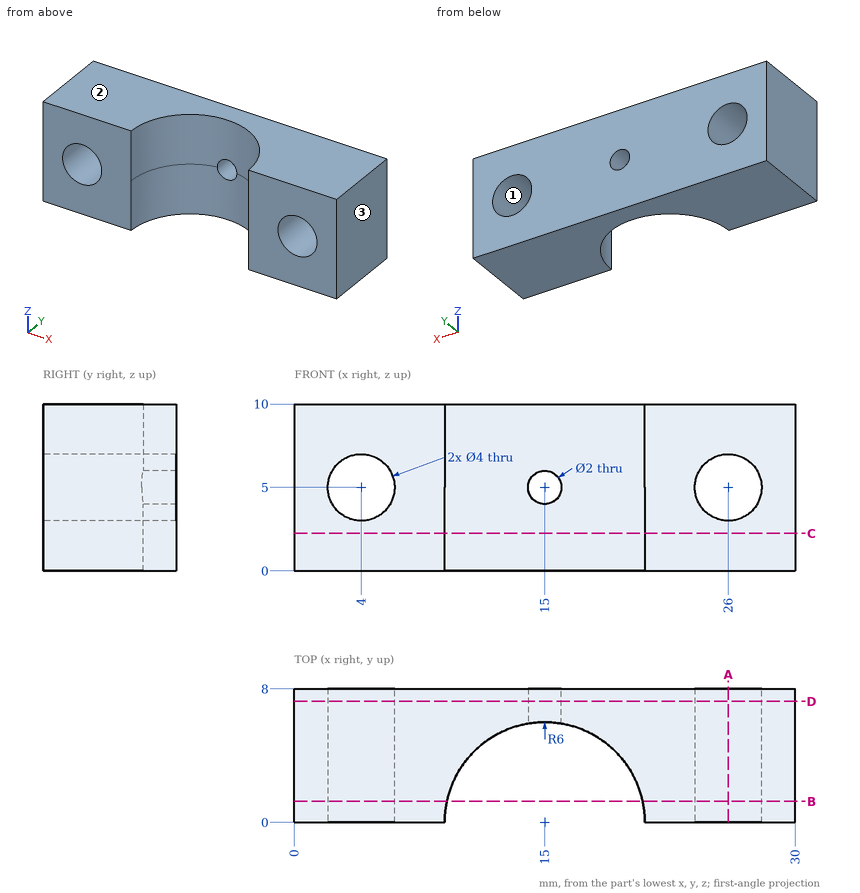
Part print with two shaded views. Sizes in mm from the minimum x, y, z corner. Round coordinates to 2 decimals unless told otherwise and drop trailing zeros. Write each loop counter-clockwise with the first axis right and the second up, starting at its lowest first coordinate (ties: lowest second). Pieces come first, ordered by that corner, then holes. Notation, with made-up numbers: (79, 64) -> (86, 64) arc R7 ccw to (86, 68) -> close; hole circle Ø1 at (84, -22). An arc over 180 degrees is marked (long way). Put each result on its own line as item: value.
Item 1: Wall check: probe 1 along Z at (x, y) = (26, 4.5); probe 2 along X at (y, z) = (6.5, 5.75); probe 3 along X at (y, z) = (7.25, 3.5). Give the ranges that are in metal, low to high. Write a range as from..to.
Here are the results:
probe 1: z = 0..3, 7..10
probe 2: x = 0..2.15, 5.85..14.34, 15.66..24.15, 27.85..30
probe 3: x = 0..2.68, 5.32..24.68, 27.32..30
Item 2: Slice it at B-B, the plane y = 1.25. Give the cut face in (x, z).
Here are the results:
outline: (0, 0) -> (9.13, 0) -> (9.13, 10) -> (0, 10) -> close; (20.87, 0) -> (30, 0) -> (30, 10) -> (20.87, 10) -> close; hole circle Ø4 at (4, 5); hole circle Ø4 at (26, 5)
Item 3: Slice it at C-C, the plane z = 2.25. Give the cut face in (x, y), plus the area to 3 significant figures.
Here are the results:
outline: (0, 0) -> (9, 0) arc R6 cw to (21, 0) -> (30, 0) -> (30, 8) -> (0, 8) -> close
area: 183 mm^2
Item 4: Flat gauge pin, fed straight in: P1, Ø2.5, axis at x = 15, z = 5, coming from the -Y side. Where does the tip first touch, or does it go through?
Here are the results:
P1: stops at y = 5.87
Item 5: Two-plate mould, pull along Z, no slides. Class the marked faces 1, 2 and 3: pulls with the +Z half, pulls with the -Z half, needs draft (parallel to the pull), parting line crosses it, or undercut.
Here are the results:
face 1: undercut
face 2: pulls with the +Z half
face 3: needs draft
Item 6: Slice it at D-D, the plane y = 7.25. Give the cut face in (x, z), plus the area to 3 significant figures.
Here are the results:
outline: (0, 0) -> (30, 0) -> (30, 10) -> (0, 10) -> close; hole circle Ø4 at (4, 5); hole circle Ø2 at (15, 5); hole circle Ø4 at (26, 5)
area: 272 mm^2
Item 7: Slice it at A-A, the plane x = 26. Give the cut face in (y, z).
Here are the results:
outline: (0, 0) -> (8, 0) -> (8, 3) -> (0, 3) -> close; (0, 7) -> (8, 7) -> (8, 10) -> (0, 10) -> close
